Autodesk Inventor part; units mm, degrees
ref_plane "YZ Plane" through (0, 0, 0) normal (1, 0, 0) x (0, 1, 0)
ref_plane "XZ Plane" through (0, 0, 0) normal (0, 1, 0) x (-1, 0, 0)
ref_plane "XY Plane" through (0, 0, 0) normal (0, 0, 1) x (1, 0, 0)
sketch "Sketch3" plane through (0, 0, 0) normal (1, 0, 0) x (0, 1, 0)
  line L0 (0, 0) -> (-75, 0)
  line L1 (-75, 0) -> (-75, -75)
  line L2 (-75, -75) -> (0, -75)
  line L3 (0, -75) -> (0, 0)
  dimension "d0" = 75
  dimension "d1" = 75
extrude "Extrusion1" add sketch "Sketch3" along normal blind 6
sketch "Sketch5" plane through (6, 0, 0) normal (1, 0, 0) x (0, 0, -1)
  circle A0 centre (12.7921, -17.6697) radius 1.5
  point P0 (0, 0)
  dimension "d27" = 3
extrude "Extrusion3" cut sketch "Sketch5" against normal blind 8.2875
equation "\"d0\" = d1"
properties part number "Reflector"
Part model, mm, in its own coordinate system. Round coordinates to 2 decimals unless told otherwise and drop trailing zeros. Write each loop counter-clockwise with the first axis right and the second up, starting at its lowest first coordinate (ties: lowest second). Pieces come first, ordered by that corner, then holes. Notation, with made-up numbers: M 13.5,-27.5 L 53.5,-27.5 A23 cw 53.5,10.5 Z; hole C -13.75,2.5 d10. An arc over 180 degrees is marked long. Return JSON: item names as keys, results as strings. Group by question number.
(1) Pin check, flat tip, straight feed: pin 1 Ø5 at (y, z) = (-17.67, -12.79) entering from -X. Stop position of the tip, or through.
(2) Drill centre lines: probe 1 along Z at (x, y) = (2.9, -17.5); probe 2 along Y at (x, z) = (5.2, -14). Where is each one in solid material? Low to high.
(3) Two-plate mould, pull along Z, no slides. Class faces 1 (the face through (3, -38, -75)), 2 (the face through (3, -75, -37)), 3 (the face through (3.042, -16.182, -12.597)): +Z half, -Z half, draft (parallel to the pull), parting line (faces both ways), or undercut.
(4) Saw through at A-A on z = -13. Write the cut outline in (x, y), then the cut area to 3 significant figures.
Returned:
{
 "1": {"pin 1": "x = 0"},
 "2": {"probe 1": "-75 to -14.28, -11.3 to 0", "probe 2": "-75 to -18.56, -16.78 to 0"},
 "3": {"face 1": "-Z half", "face 2": "draft", "face 3": "undercut"},
 "4": {"outline": "M 0,-75 L 6,-75 L 6,-19.16 L 0,-19.16 Z; M 0,-16.18 L 6,-16.18 L 6,0 L 0,0 Z", "area": "432 mm²"}
}
